```python
from build123d import *

# Parameters (mm, degrees)
PLATE_THICKNESS_3MM_DEPTH = 3
SKETCH_1_W                = 0.35
SKETCH_1_H                = 60
SKETCH_1_H_2              = 20
CUT_EXTRUDE_1_DEPTH       = 3


with BuildPart() as part:
    # Sketch1 → Plate_thickness_3mm (new body)
    with BuildSketch(Plane.XY):
        Polygon((28.57, 0), (0, 0), (0, 20), (3, 20), (3, 40), (0, 40), (0, 60), (14.285, 60), (14.285, 63), (17.285, 63), (17.285, 60), (28.57, 60), (28.57, 40), (31.57, 40), (31.57, 20), (28.57, 20), align=None)
    extrude(amount=PLATE_THICKNESS_3MM_DEPTH)

    # 草图1 → 切除-拉伸1 (cut)
    with BuildSketch(Plane.XY.offset(3)):
        with Locations((0.175, 30)):
            Rectangle(SKETCH_1_W, SKETCH_1_H)
        with Locations((3.175, 30)):
            Rectangle(SKETCH_1_W, SKETCH_1_H_2)
        with Locations((28.395, 50)):
            Rectangle(SKETCH_1_W, SKETCH_1_H_2)
        with Locations((31.395, 30)):
            Rectangle(SKETCH_1_W, SKETCH_1_H_2)
        with Locations((28.395, 10)):
            Rectangle(SKETCH_1_W, SKETCH_1_H_2)
    extrude(amount=-CUT_EXTRUDE_1_DEPTH, mode=Mode.SUBTRACT)


solid = part.part
```
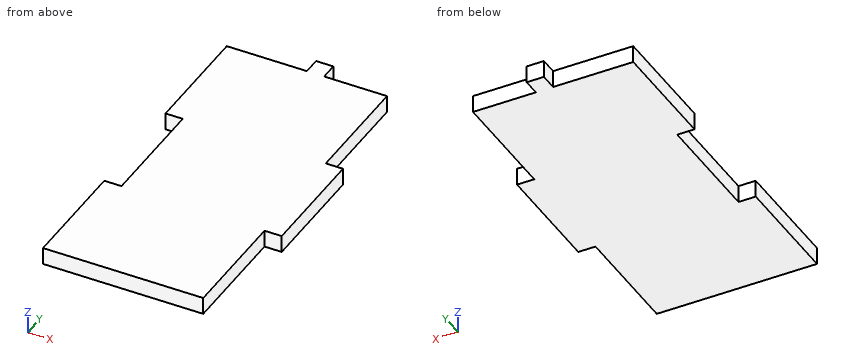
The model under review builds one solid part; all positions refer to its coordinate system, in mm. Give positions to 0.01 mm unless a question says otherwise; leave off trailing zeros. Loops run counter-clockwise (first coordinate to the right, second up) from the corner with the lowest first, then second, coordinate; pieces in that order, holes last. Notation, with made-up numbers: (8.5, -17.75) - (51.5, -17.75) arc R24 cw to (51.5, 3.25) - close; hole circle Ø3 at (66.25, 28). An arc over 180 degrees is marked (long way). Answer as a JSON object with one key per item and string values.
Q1. Add section B-B on y = 22. State the section outline as (x, z) points.
Worked out:
{"outline": "(3.35, 0) - (31.22, 0) - (31.22, 3) - (3.35, 3) - close"}
Q2. Add section A-A on z = 2.25. State the section outline as (x, y) points (3 decimals), plus the area to 3 significant figures.
Worked out:
{"outline": "(0.35, 0) - (28.22, 0) - (28.22, 20) - (31.22, 20) - (31.22, 40) - (28.22, 40) - (28.22, 60) - (17.285, 60) - (17.285, 63) - (14.285, 63) - (14.285, 60) - (0.35, 60) - (0.35, 40) - (3.35, 40) - (3.35, 20) - (0.35, 20) - close", "area": "1,680 mm^2"}
Q3. Insertion check: pin 1 (0.9 mm diameter, centred on y = 52, z = 2, fed in from +X); pin 2 (1.5 mm diameter, centred on x = 21, z = 1.5, fed in from +Y); pin 3 (1.5 mm diameter, centred on x = 30, z = 1, fed in from +Y). Each pin has a flat end and moves straight along its axis. Give the tip position at first contact, or say it passes through.
Worked out:
{"pin 1": "stops at x = 28.22", "pin 2": "stops at y = 60", "pin 3": "stops at y = 40"}
Q4. To check wall thickness, follow line 1 along Y through (x, z) = (28, 1.6); line 2 along X through (y, z) = (26, 1.6); line 3 along Y through (x, z) = (29, 2.75). State the ranges of each line that lie inside material, in increasing order.
Worked out:
{"line 1": "y = 0 to 60", "line 2": "x = 3.35 to 31.22", "line 3": "y = 20 to 40"}
Q5. Add section C-C on x = 10. State the section outline as (y, z) points, plus the area to 3 significant figures.
Worked out:
{"outline": "(0, 0) - (60, 0) - (60, 3) - (0, 3) - close", "area": "180 mm^2"}
